from build123d import *

# Parameters (mm, degrees)
F0_W     = 100
F0_H     = 100
F1_DEPTH = 50


with BuildPart() as f1:
    # F0 (on Top) → F1 (new body, symmetric)
    with BuildSketch(Plane.XY):
        Rectangle(F0_W, F0_H)
    extrude(amount=F1_DEPTH, both=True)

    # F2 (on Top) → F3 (revolve, cut)
    with BuildSketch(Plane.XY):
        Polygon((75, 0), (50, 0), (75, -75), align=None)
    revolve(axis=Axis((0, -37.5, 0), (0, -1, 0)), mode=Mode.SUBTRACT)


solid = f1.part
Check sheet for the modelled part. Datum: model origin and axes. Units: mm. A direction names the side the tool comes from. Round coordinates to 2 decimals unless told otherwise and drop trailing zeros. Loops run counter-clockwise (first coordinate to the right, second up) from the corner with the lowest first, then second, coordinate; pieces in that order, holes last. Notation, with made-up numbers: (8, 17) -> (54, 17) arc R30 cw to (54, 51) -> close; hole circle Ø1 at (-6, -1.5). An arc over 180 degrees is marked (long way). Put each result on its own line as item: value. Start each with the question number.
1. Access from +Z, -Z, +X, -X, +Y, -Y to the whole of each face (thin tool, end or side, straight path). Record for faces 4 (the face through (-40, 0, -38)), 5 (the face through (50, -31, 1)).
2. Section check B-B (y = -4). Enter the section's corners in (x, z).
3. Gauge pin test, flat ends, axial feed: pin 1 (3 mm diameter, centred on x = -28, y = -5, fed in from -Z); pin 2 (3 mm diameter, centred on x = -38.5, y = -26.5, fed in from -Z). Record the tip position at first contact, or that the pin passes through.
4. Draft check along Y on faces 1 (the face through (-50, -31, 1)), 2 (the face through (-1, -50, 1)), 3 (the face through (-40, 0, 38)). Enter one of: +Y half, -Y half, draft (parallel to the pull), parting line (faces both ways), or undercut.
5. Section check A-A (y = -28). Enter the section's corners in (x, z).
6. Scan lines: probe 1 along Z at (x, y) = (33, -18); probe 2 along Z at (x, y) = (-43, -29). Record each from-to range of solid material in increasing order.
Findings:
1. face 4: -Z, -X
1. face 5: +Z, -Z, +X, +Y, -Y
2. outline: (-50, -11.62) arc R51.33 ccw to (-11.62, -50) -> (11.62, -50) arc R51.33 ccw to (50, -11.62) -> (50, 11.62) arc R51.33 ccw to (11.62, 50) -> (-11.62, 50) arc R51.33 ccw to (-50, 11.62) -> close
3. pin 1: stops at z = -44.53
3. pin 2: stops at z = -45.9
4. face 1: draft
4. face 2: -Y half
4. face 3: undercut
5. outline: (-50, -31.94) arc R59.33 ccw to (-31.94, -50) -> (31.94, -50) arc R59.33 ccw to (50, -31.94) -> (50, 31.94) arc R59.33 ccw to (31.94, 50) -> (-31.94, 50) arc R59.33 ccw to (-50, 31.94) -> close
6. probe 1: z = -45.24 to 45.24
6. probe 2: z = -41.37 to 41.37
